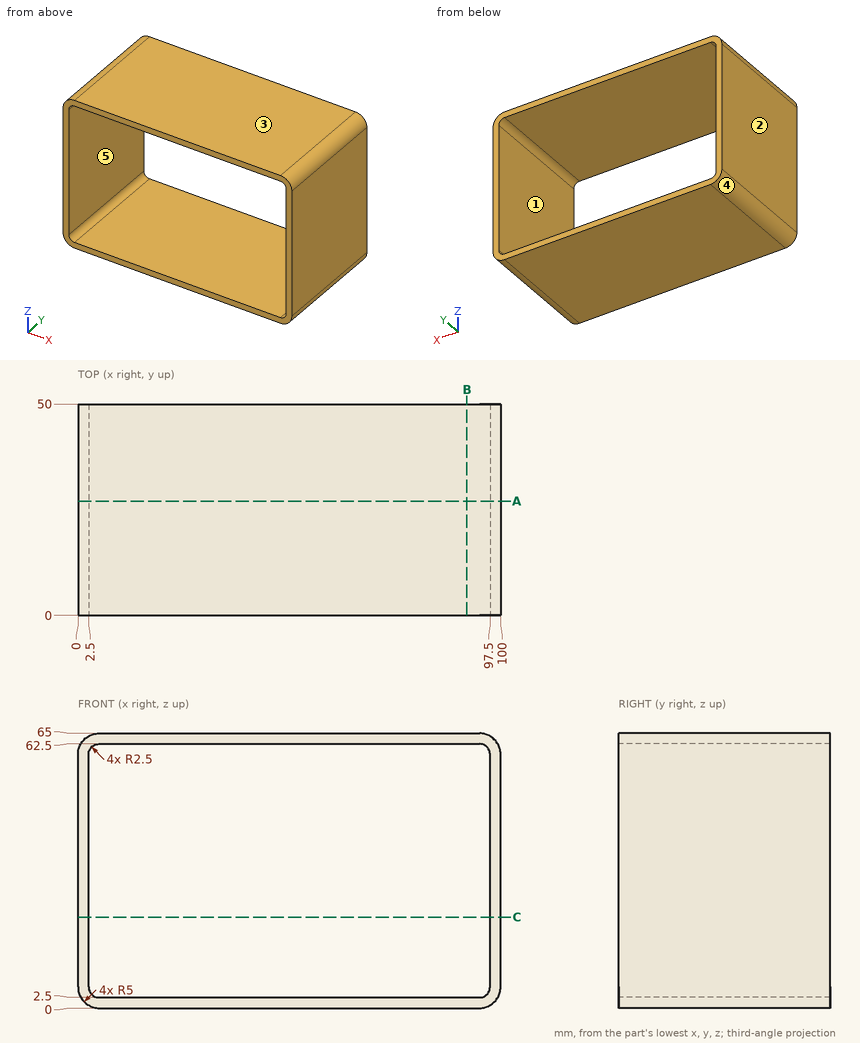
Design review of the part shown in the three views and the two pictorial views. Dimensions are in mm from the part's minimum x, y and z. A direction names the side the tool comes from. Give positions to 0.01 mm unless a question says otherwise; leave off trailing zeros. Loops run counter-clockwise (first coordinate to the right, second up) from the corner with the lowest first, then second, coordinate; pieces in that order, holes last. Notation, with made-up numbers: M 60,8 L 71,8 A21 ccw 71,12 Z; hole C -38.5,78 d10. An arc over 180 degrees is marked long. Put each result on its own line as item: value. Start each with the question number.
(1) Machinability: for the marked faces 4 and 5, which of the approach directions +Z, -Z, +X, -X, +Y, -Y give a long, thin tool a straight path to every point of the face, cutting with its end or side? Answer none if there is none.
(2) Add section A-A, the plane y = 27. Write out the cut boundary in (x, z), then the cut area to 3 significant figures.
(3) Add section C-C, the plane z = 21.5. Write out the cut boundary in (x, y).
(4) Wall thickness on L1, parallel to Z at x = 32, y = 38; L2, parallel to X at y = 22, z = 51; L3, parallel to X at y = 26, z = 4: over which ranges is each line inside the solid? List them lowest first.
(5) The part is to be moulded in two halves that separate along Z. For the marked faces 1, 2 and 3, say which applies: +Z half, -Z half, draft (parallel to the pull), parting line (faces both ways), or undercut.
(6) Add section B-B, the plane x = 92. Write out the cut boundary in (y, z).
(7) For pin 1 (8 mm diameter, centred on y = 41.5, z = 54, fed in from -X), flat-tipped, find the tip position at first contact; note if it passes through.
Result:
1. face 4: -Z, -X, +Y, -Y
1. face 5: +Y, -Y
2. outline: M 0,5 A5 ccw 5,0 L 95,0 A5 ccw 100,5 L 100,60 A5 ccw 95,65 L 5,65 A5 ccw 0,60 Z; hole M 2.5,5 A2.5 ccw 5,2.5 L 95,2.5 A2.5 ccw 97.5,5 L 97.5,60 A2.5 ccw 95,62.5 L 5,62.5 A2.5 ccw 2.5,60 Z
2. area: 784 mm^2
3. outline: M 0,0 L 2.5,0 L 2.5,50 L 0,50 Z; M 97.5,0 L 100,0 L 100,50 L 97.5,50 Z
4. L1: z = 0 to 2.5, 62.5 to 65
4. L2: x = 0 to 2.5, 97.5 to 100
4. L3: x = 0.1 to 2.71, 97.29 to 99.9
5. face 1: undercut
5. face 2: draft
5. face 3: +Z half
6. outline: M 0,0 L 50,0 L 50,2.5 L 0,2.5 Z; M 0,62.5 L 50,62.5 L 50,65 L 0,65 Z
7. pin 1: stops at x = 0
